Can you work these out from the model? Positions are in its coordinate system, mm. Face numbers are marked on the shaded views. A direction names the side the tool comes from. Give positions to 0.01 mm unless a question says otherwise; leave off trailing zeros. Loops run counter-clockwise (first coordinate to the right, second up) from the corner with the lowest first, then second, coordinate; pieces in that order, holes last. Notation, with made-up numbers: (-3.5, 76) - (34.5, 76) arc R14 cw to (34.5, 96) - close; hole circle Ø9 at (23, 9). An arc over 180 degrees is marked (long way). Answer in a Markdown table with one row per item.
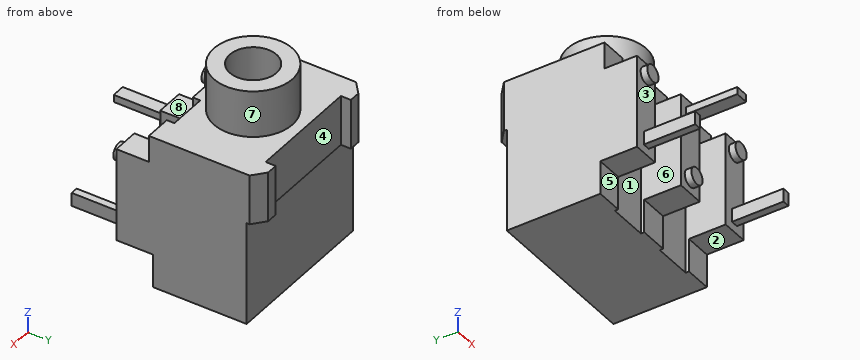
from build123d import *

# Parameters (mm, degrees)
EXTRUDE2_DEPTH     = 6.35
SKETCH3_OUTSIDE_W  = 18.79
SKETCH3_OUTSIDE_H  = 17.063
CUT_EXTRUDE1_DEPTH = 18.24066982
SKETCH6_R          = 2.9845
SKETCH6_R_2        = 1.778
EXTRUDE4_DEPTH     = 3.556
SKETCH7_R          = 0.635
EXTRUDE5_DEPTH     = 0.508
SKETCH8_W          = 1.016
SKETCH8_H          = 0.5588
SKETCH8_W_2        = 0.5588
SKETCH8_H_2        = 1.016
EXTRUDE6_DEPTH     = 3.9116


with BuildPart() as part:
    # Sketch2 → Extrude2 (new, symmetric)
    with BuildSketch(Plane(origin=(0, 0, 0), x_dir=(0, 0, -1), z_dir=(1, 0, 0))):
        Polygon((2.032, 0), (9.144, 0), (9.144, 2.794), (11.684, 2.794), (11.684, 9.906), (3.81, 9.906), (3.81, 10.9728), (0, 10.9728), (0, 2.471612931), (2.032, 2.471612931), align=None)
    extrude(amount=EXTRUDE2_DEPTH, both=True)

    # Sketch3 outside → Cut-Extrude1 (cut, through all)
    with BuildSketch(Plane.XY):
        with Locations((0, 5.4865)):
            Rectangle(SKETCH3_OUTSIDE_W, SKETCH3_OUTSIDE_H)
        Polygon((-4.011698259, 0), (-6.0452, 0), (-6.0452, 10.128452415), (-5.112567083, 10.922), (-4.2672, 10.922), (-4.2672, 10.16), (4.2672, 10.16), (4.2672, 10.922), (5.112567083, 10.922), (6.0452, 10.128452415), (6.0452, 0), (4.011698259, 0), (4.011698259, 3.048), (1.0668, 3.048), (1.0668, 0), (-1.0668, 0), (-1.0668, 3.048), (-4.011698259, 3.048), align=None, mode=Mode.SUBTRACT)
    extrude(amount=-CUT_EXTRUDE1_DEPTH, mode=Mode.SUBTRACT)

    # Sketch6 → Extrude4 (add)
    with BuildSketch(Plane.XY):
        with Locations(Location((0, 6.35, 0), (0, 0, 90))):
            Circle(SKETCH6_R)
        with Locations((0, 6.35)):
            Circle(SKETCH6_R_2, mode=Mode.SUBTRACT)
    extrude(amount=EXTRUDE4_DEPTH)

    # Sketch7 → Extrude5 (add)
    with BuildSketch(Plane(origin=(0, 0, 0), x_dir=(1, 0, 0), z_dir=(0, 1, 0))):
        with Locations(Location((0, 8.001, 0), (0, 0, 270))):
            Circle(SKETCH7_R)
        with Locations(Location((5.0038, 2.9972, 0), (0, 0, 270))):
            Circle(SKETCH7_R)
        with Locations(Location((-5.0038, 2.9972, 0), (0, 0, 270))):
            Circle(SKETCH7_R)
    extrude(amount=-EXTRUDE5_DEPTH)

    # Sketch8 → Extrude6 (add)
    with BuildSketch(Plane(origin=(0, 0, 0), x_dir=(1, 0, 0), z_dir=(0, 1, 0))):
        with Locations((0, 2.9972)):
            Rectangle(SKETCH8_W, SKETCH8_H)
        with Locations((-5.0038, 8.001)):
            Rectangle(SKETCH8_W_2, SKETCH8_H_2)
        with Locations((5.0038, 8.001)):
            Rectangle(SKETCH8_W_2, SKETCH8_H_2)
    extrude(amount=-EXTRUDE6_DEPTH)


solid = part.part
Q1. Imagine slicing it at D-D, the plane y = 6.35. Write out the boundary of the cut face in (x, z).
Checked values:
| item | result |
|---|---|
| outline | (-6.05, -11.68) - (6.05, -11.68) - (6.05, 0) - (2.98, 0) - (2.98, 3.56) - (1.78, 3.56) - (1.78, 0) - (-1.78, 0) - (-1.78, 3.56) - (-2.98, 3.56) - (-2.98, 0) - (-6.05, 0) - close |
Q2. If we mould it in two halves opening along Z, with no side actions, what happens to the marked faces 1, 2 and 3? For each: released by +Z, released by -Z, zero draft, split by the parting line, or undercut.
Checked values:
| item | result |
|---|---|
| face 1 | zero draft |
| face 2 | released by -Z |
| face 3 | undercut |
Q3. Imagine slicing it at C-C, the plane x = 0. Write out the boundary of the cut face in (y, z), and give its area (3 significant figures).
Checked values:
| item | result |
|---|---|
| outline | (-3.91, -3.28) - (0, -3.28) - (0, -7.37) - (-0.51, -7.37) - (-0.51, -8.64) - (0, -8.64) - (0, -9.14) - (2.79, -9.14) - (2.79, -11.68) - (9.91, -11.68) - (9.91, -3.81) - (10.16, -3.81) - (10.16, 0) - (9.33, 0) - (9.33, 3.56) - (8.13, 3.56) - (8.13, 0) - (4.57, 0) - (4.57, 3.56) - (3.37, 3.56) - (3.37, 0) - (2.47, 0) - (2.47, -2.03) - (0, -2.03) - (0, -2.72) - (-3.91, -2.72) - close |
| area | 116 mm² |
Q4. On a 3-axis mill with a long thin cutter (end or side, diameter ignored), from which of +Z, -Z, +X, -X, +Y, -Y can I reach the whole of each face in a straight line? I mean the marked faces 4, 5, 6, 7 and 8. Say none if no direction works.
Checked values:
| item | result |
|---|---|
| face 4 | +Z, -Z, +Y |
| face 5 | -Z, +X, -X, -Y |
| face 6 | +Z, -Z, -Y |
| face 7 | +Z |
| face 8 | +Z, +X, -X, -Y |
Q5. Imagine slicing it at A-A, the plane y = 1. Write out the boundary of the cut face in (x, z).
Checked values:
| item | result |
|---|---|
| outline | (-6.05, -9.14) - (-4.01, -9.14) - (-4.01, -2.03) - (-6.05, -2.03) - close; (-1.07, -9.14) - (1.07, -9.14) - (1.07, -2.03) - (-1.07, -2.03) - close; (4.01, -9.14) - (6.05, -9.14) - (6.05, -2.03) - (4.01, -2.03) - close |
Q6. Imagine slicing it at B-B, the plane z = -8. Write out the boundary of the cut face in (x, y) (3 decimals).
Checked values:
| item | result |
|---|---|
| outline | (-6.045, 0) - (-5.283, 0) - (-5.283, -3.912) - (-4.724, -3.912) - (-4.724, 0) - (-4.012, 0) - (-4.012, 3.048) - (-1.067, 3.048) - (-1.067, 0) - (-0.635, 0) - (-0.635, -0.508) - (0.635, -0.508) - (0.635, 0) - (1.067, 0) - (1.067, 3.048) - (4.012, 3.048) - (4.012, 0) - (4.724, 0) - (4.724, -3.912) - (5.283, -3.912) - (5.283, 0) - (6.045, 0) - (6.045, 9.906) - (-6.045, 9.906) - close |
Q7. If I drill on line 1 (Z direction, x = 0, y = 3); line 2 (Y direction, x = -1.5, z = 1); line 3 (Y direction, x = -3.5, z = -8.25), over which ranges is the centre line in solid material (lowest first)? Write a range as [from, to].
Checked values:
| item | result |
|---|---|
| line 1 | z = [-11.68, 0] |
| line 2 | y = [3.77, 5.4], [7.3, 8.93] |
| line 3 | y = [3.05, 9.91] |
Q8. For pin 1 (0.8 mm diameter, centred on x = 0, y = -2, fed in from +Z); pin 2 (3 mm diameter, centred on x = -4.5, z = -2, fed in from -Y); pin 3 (0.6 mm diameter, centred on x = 0, z = -4.5, fed in from -Y); pin 4 (1.5 mm diameter, centred on x = -2, y = 0, fed in from -Z), each with a flat end and sliding along its axis, tell me the tip position at first contact or that it passes through.
Checked values:
| item | result |
|---|---|
| pin 1 | stops at z = -2.72 |
| pin 2 | stops at y = -0.51 |
| pin 3 | stops at y = 0 |
| pin 4 | passes through |
